Verification items for the finished model (mm, model axes). A direction names the side the tool comes from. Coordinates: 2 decimals unless noted, no trailing zeros. Loops run counter-clockwise (first coordinate to the right, second up) from the corner with the lowest first, then second, coordinate; pieces in that order, holes last. Notation, with made-up numbers: (15, 85.25) -> (35, 85.25) arc R11 ccw to (35, 95.25) -> close; hole circle Ø9 at (2, 37). An arc over 180 degrees is marked (long way). Write item = value, one per line.
```python
from build123d import *

# Parameters (mm, degrees)
F0_R     = 152.4
F1_DEPTH = 12.7
F2_R     = 12.7
F3_DEPTH = 101.6
F4_R     = 6.35
F5_DEPTH = 76.2
F6_COUNT = 3


with BuildPart() as f1:
    # F0 (on Top) → F1 (new body)
    with BuildSketch(Plane.XY):
        Circle(F0_R)
    extrude(amount=F1_DEPTH)

    # F2 (on face) → F3 (join)
    with BuildSketch(Plane.XY.offset(12.7)):
        Circle(F2_R)
    extrude(amount=F3_DEPTH)

    # F4 (on face) → F5 (join)
    with BuildSketch(Plane.XY.offset(12.7)):
        with Locations((0, 127)):
            Circle(F4_R)
    extrude(amount=F5_DEPTH)

    # F6: F1 ×3 about axis
    f6_axis = Axis((0, 0, 12.7), (0, 0, -1))


with BuildPart() as f1_1:
    add(f1.part)
    for i in range(1, F6_COUNT):
        add(f1.part.rotate(f6_axis, i * 360 / F6_COUNT))


solid = f1_1.part
```
1) Sectioned sample at A-A, the plane x = 0. Record the cut outline in (y, z).
Ans:
outline = (-152.4, 0) -> (152.4, 0) -> (152.4, 12.7) -> (133.35, 12.7) -> (133.35, 88.9) -> (120.65, 88.9) -> (120.65, 12.7) -> (12.7, 12.7) -> (12.7, 114.3) -> (-12.7, 114.3) -> (-12.7, 12.7) -> (-152.4, 12.7) -> close
2) Sectioned sample at B-B, the plane y = 0. Record the cut outline in (x, z).
Ans:
outline = (-152.4, 0) -> (152.4, 0) -> (152.4, 12.7) -> (12.7, 12.7) -> (12.7, 114.3) -> (-12.7, 114.3) -> (-12.7, 12.7) -> (-152.4, 12.7) -> close
3) Depth check by flat-ended pin: pin 1 Ø10 at (x, y) = (-111, -63) entering from +Z; pin 2 Ø10 at (x, y) = (-60.5, -27.5) entering from +Z. Enter the tip coordinate at first touch or a pass-through.
Ans:
pin_1 = 88.9
pin_2 = 12.7
4) Sectioned sample at D-D, the plane z = 46. Record the cut outline in (x, y).
Ans:
outline = circle Ø12.7 at (-109.99, -63.5); circle Ø25.4 at (0, 0); circle Ø12.7 at (0, 127); circle Ø12.7 at (109.99, -63.5)
5) Tool access check on faces 4 (the face through (32, 2, 12.7)), 5 (the face through (0, 127, 88.9)), 6 (the face through (110, -63, 88.9)). Record the directions out of +Z, -Z, +X, -X, +Y, -Y that give a thin tool (end or side, any length) a straight path to the whole face; none if there is none.
Ans:
face_4 = +Z
face_5 = +Z, +X, -X, +Y
face_6 = +Z, +X, -X, +Y, -Y
6) Sectioned sample at C-C, the plane z = 9. Record the cut outline in (x, y), plus the area to 3 significant figures.
Ans:
outline = circle Ø304.8 at (0, 0)
area = 73,000 mm2
7) Release check for a two-part mould opening along X. For faces 1 (the face through (-106.572, -58.146, 50.267)), 2 (the face through (0, 0, 114.3)), 3 (the face through (-2.75, -12.4, 62.79)) record: pulls with the +X half, pulls with the -X half, needs draft (parallel to the pull), parting line crosses it, or undercut.
Ans:
face_1 = undercut
face_2 = needs draft
face_3 = parting line crosses it
8) Material ranges on line 1 (Z direction, x = 77, y = 115.5); line 2 (X direction, y = -27, z = 8.5); line 3 (X direction, y = -66.5, z = 28), recorded low to high.
Ans:
line_1 = 0 to 12.7
line_2 = -149.99 to 149.99
line_3 = -115.58 to -104.39, 104.39 to 115.58
